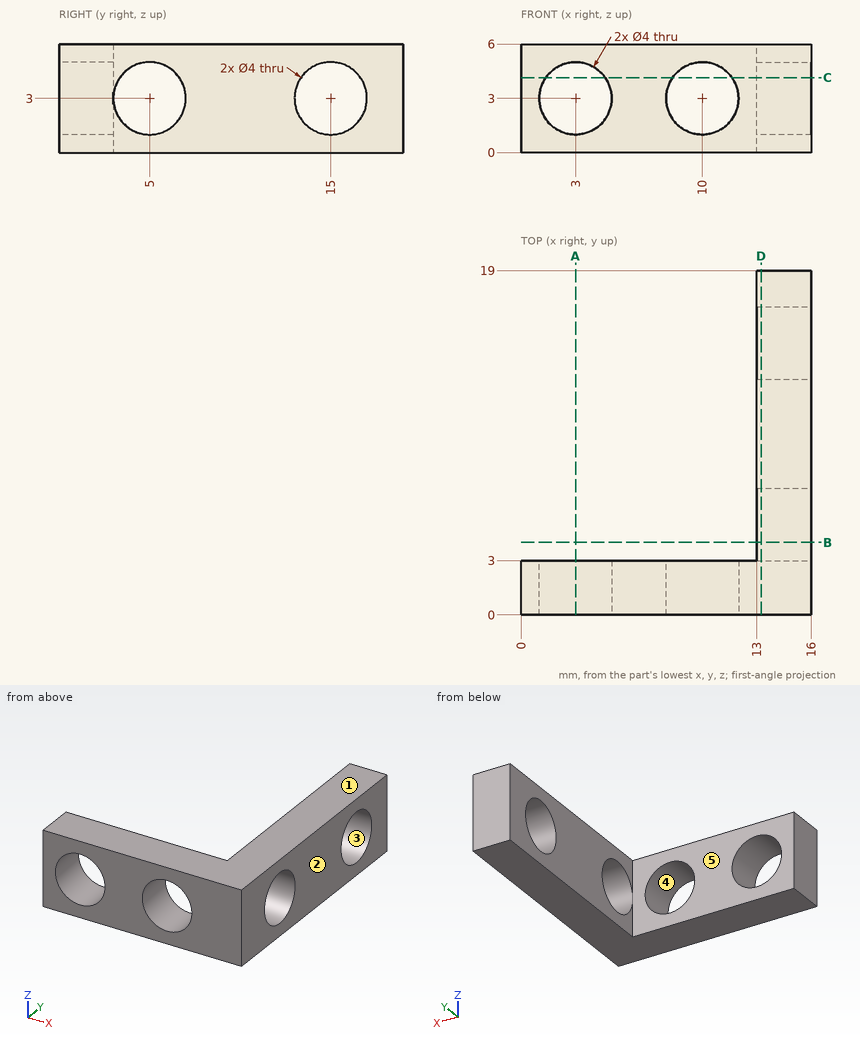
Print and shaded views of the part. All mm, measured from the part's lowest x, y and z. A direction names the side the tool comes from. Give positions to 0.01 mm unless a question says otherwise; leave off trailing zeros. Loops run counter-clockwise (first coordinate to the right, second up) from the corner with the lowest first, then second, coordinate; pieces in that order, holes last.
1) Wall check: line 1 (Y direction, x = 14.85, z = 3); line 2 (X direction, y = 1.9, z = 3); line 3 (Z direction, x = 10, y = 2). Give the ranges that are in metal, low to high.
2) Tool access for the marked faces 4 and 5: list every direction of +Z, -Z, +X, -X, +Y, -Y with a clear straight run to the whole face (end or side of a thin tool).
3) Flat gauge pins, fed straight in: pin 1 Ø3 at (y, z) = (12, 2) entering from -X; pin 2 Ø3 at (x, z) = (8.5, 3) entering from +Y. Where does each tip first touch, or does it go through?
4) Pull direction Z, two halves, no side cores. Call the marked faces 1, 2 and 3: +Z half, -Z half, draft (parallel to the pull), parting line (faces both ways), or undercut.
5) Saw through at B-B (y = 4). Write the cut outline in (x, z).
6) Saw through at D-D (x = 13.25). Write the cut outline in (y, z), plus the area to 3 significant figures.
7) Saw through at C-C (z = 4.15). Write the cut outline in (x, y), plus the area to 3 significant figures.
8) Saw through at A-A (x = 3). Write the cut outline in (y, z).
Answer block:
1. line 1: y = 0 to 3, 7 to 13, 17 to 19
1. line 2: x = 0 to 1, 5 to 8, 12 to 16
1. line 3: z = 0 to 1, 5 to 6
2. face 4: +Y, -Y
2. face 5: +Z, -Z, -X, +Y
3. pin 1: stops at x = 13
3. pin 2: stops at y = 3
4. face 1: +Z half
4. face 2: draft
4. face 3: undercut
5. outline: (13, 0) - (16, 0) - (16, 1.27) - (13, 1.27) - close; (13, 4.73) - (16, 4.73) - (16, 6) - (13, 6) - close
6. outline: (0, 0) - (19, 0) - (19, 6) - (0, 6) - close; hole circle Ø4 at (5, 3); hole circle Ø4 at (15, 3)
6. area: 88.9 mm2
7. outline: (0, 0) - (1.36, 0) - (1.36, 3) - (0, 3) - close; (4.64, 0) - (8.36, 0) - (8.36, 3) - (4.64, 3) - close; (11.64, 0) - (16, 0) - (16, 3.36) - (13, 3.36) - (13, 3) - (11.64, 3) - close; (13, 6.64) - (16, 6.64) - (16, 13.36) - (13, 13.36) - close; (13, 16.64) - (16, 16.64) - (16, 19) - (13, 19) - close
7. area: 56.7 mm2
8. outline: (0, 0) - (3, 0) - (3, 1) - (0, 1) - close; (0, 5) - (3, 5) - (3, 6) - (0, 6) - close
